Input: part model. Units: mm. Frame: model coordinates. Face numbers are marked on the shaded views. Coordinates: 2 decimals unless noted, no trailing zeros. Order: outer loops, then holes, each group sorted by start corner. A loop starts at its lowest first (then second) coordinate and runs counter-clockwise, first axis right, second up. Notation, with made-up numbers: (38, 89.5) -> (93, 89.5) arc R21 cw to (93, 106.5) -> close; hole circle Ø5 at (16.5, 51). An arc over 180 degrees is marked (long way). Answer as CSV lines item,"result".
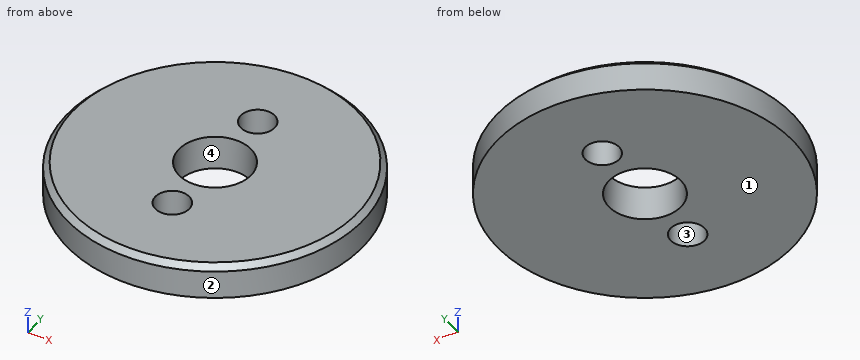
from build123d import *

# Parameters (mm, degrees)
SKETCH_1_R      = 13
SKETCH_1_R_2    = 3.175
SKETCH_1_R_3    = 1.494405319
EXTRUDE_1_DEPTH = 3
CHAMFER_1_SIZE  = 0.5


with BuildPart() as part:
    # Эскиз1 → Вытянуть1 (new body)
    with BuildSketch(Plane.XY):
        Circle(SKETCH_1_R)
        Circle(SKETCH_1_R_2, mode=Mode.SUBTRACT)
        with Locations((0, 6)):
            Circle(SKETCH_1_R_3, mode=Mode.SUBTRACT)
        with Locations((0, -6)):
            Circle(SKETCH_1_R_3, mode=Mode.SUBTRACT)
    extrude(amount=EXTRUDE_1_DEPTH)

    # Фаска1
    chamfer_1_edges = [part.edges().sort_by_distance(p)[0] for p in [
        (-13, 0, 3),
    ]]
    chamfer(chamfer_1_edges, length=CHAMFER_1_SIZE)


solid = part.part
1. Cut plane B-B (z = 1.05). Return the cut outline in (x, y) (3 decimals).
Findings:
outline,"circle Ø26 at (0, 0); hole circle Ø6.35 at (0, 0); hole circle Ø2.989 at (0, -6); hole circle Ø2.989 at (0, 6)"
2. Contact query for flat-ended pins moving along their axis: pin 1 (6 mm diameter, centred on x = 2.5, y = -9, fed in from -Z); pin 2 (1.5 mm diameter, centred on y = -4.5, z = 1.5, fed in from +X); pin 3 (5.5 mm diameter, centred on x = 0, y = 0, fed in from +Z); pin 4 (1.5 mm diameter, centred on x = -1.5, z = 0.5, fed in from -Y). Output: stop coordinate, or through.
Findings:
pin 1,"stops at z = 0"
pin 2,"stops at x = 12.45"
pin 3,"passes through"
pin 4,"stops at y = -12.98"
3. Mould query, pull axis X, two halves, no side actions, for the marked faces 1, 2, 3 and 4. Classes: released by +X, released by -X, zero draft, split by the parting line, or undercut.
Findings:
face 1,"zero draft"
face 2,"split by the parting line"
face 3,"undercut"
face 4,"undercut"
4. Ray query, line 1 along Y through (x, z) = (0, 1.4) (3 decimals); line 2 along Y through (x, z) = (-2.25, 0.8); line 3 along X through (y, z) = (6.75, 1.5). Return the intervals inside material, ascending.
Findings:
line 1,"y = -13 to -7.494, -4.506 to -3.175, 3.175 to 4.506, 7.494 to 13"
line 2,"y = -12.8 to -2.24, 2.24 to 12.8"
line 3,"x = -11.11 to -1.29, 1.29 to 11.11"
5. Cut plane A-A (x = 0). Return the cut outline in (y, z) (3 decimals), plus the area to 3 significant figures.
Findings:
outline,"(-13, 0) -> (-7.494, 0) -> (-7.494, 3) -> (-12.5, 3) -> (-13, 2.5) -> close; (-4.506, 0) -> (-3.175, 0) -> (-3.175, 3) -> (-4.506, 3) -> close; (3.175, 0) -> (4.506, 0) -> (4.506, 3) -> (3.175, 3) -> close; (7.494, 0) -> (13, 0) -> (13, 2.5) -> (12.5, 3) -> (7.494, 3) -> close"
area,"40.8 mm2"
